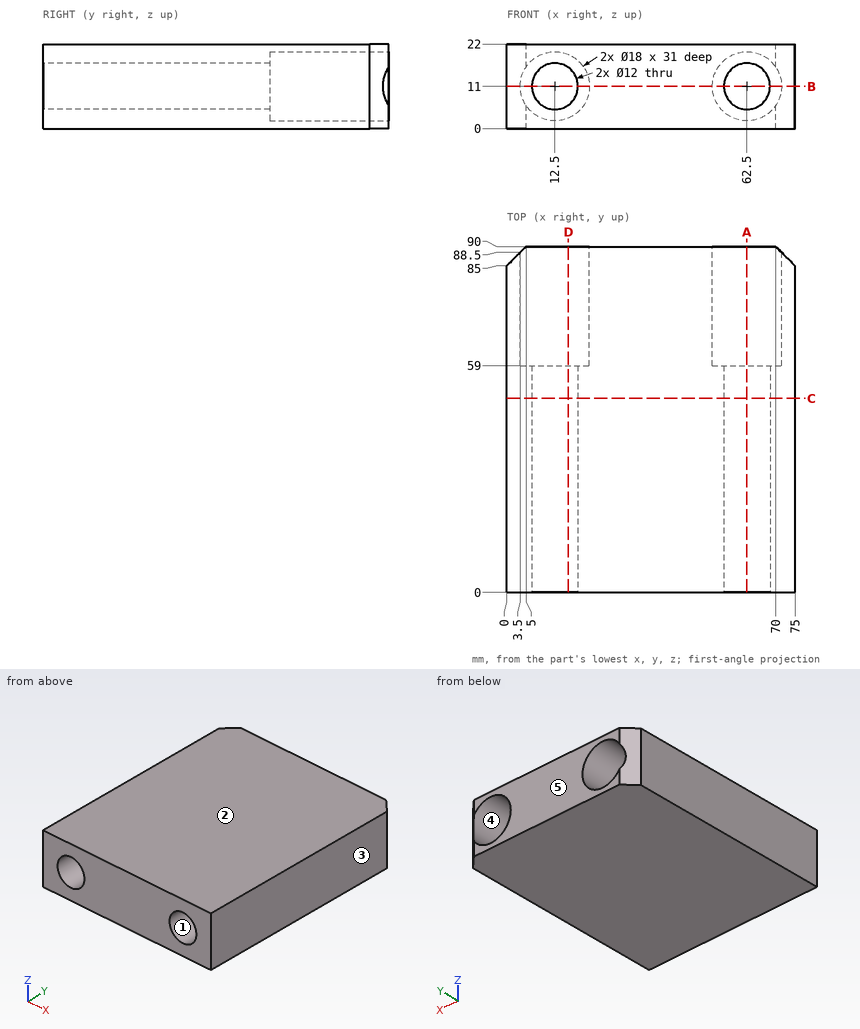
Design review of the part shown in the three views and the two pictorial views. Dimensions are in mm from the part's minimum x, y and z. A direction names the side the tool comes from. Round coordinates to 2 decimals unless told otherwise and drop trailing zeros. Write each loop counter-clockwise with the first axis right and the second up, starting at its lowest first coordinate (ties: lowest second). Pieces come first, ordered by that corner, then holes. Notation, with made-up numbers: (24, -18) - (49, -18) arc R35 cw to (49, 15) - close; hole circle Ø9 at (-17.5, 40). An arc over 180 degrees is marked (long way). Write item = value, one per line. Start each with the question number.
1. For pin 1 Ø7 at (x, z) = (62.5, 11) entering from +Y; pin 2 Ø9 at (x, z) = (11, 13.5) entering from +Y, all flat-tipped, find the tip position at first contact; note any pin that passes through.
2. Consider section A-A on x = 62.5. State the section outline as (y, z) points.
3. For the marked faces 4 and 5, list the 3-axis set-ups (+Z, -Z, +X, -X, +Y, -Y) from which the entire face can be reached by the end or side of a thin tool; tool diameter is ignored.
4. Consider section C-C on y = 50.5. State the section outline as (x, z) points, plus the area to 3 significant figures.
5. Wall thickness on L1, parallel to X at y = 25, z = 10.75; L2, parallel to X at y = 78, z = 11; L3, parallel to Z at x = 62, y = 36: over which ranges is each line inside the solid? List them lowest first.
6. Draft analysis for pull direction X (two halves, no side actions). For the marked faces 1, 2 and 3, state which applies: released by +X, released by -X, zero draft, split by the parting line, or undercut.
7. Consider section D-D on x = 16. State the section outline as (y, z) points.
8. Consider section B-B on z = 11. State the section outline as (x, y) points, plus the area to 3 significant figures.
Evaluation:
q1.pin_1 = through
q1.pin_2 = 59
q2.outline = (0, 0) - (90, 0) - (90, 2) - (59, 2) - (59, 5) - (0, 5) - close; (0, 17) - (59, 17) - (59, 20) - (90, 20) - (90, 22) - (0, 22) - close
q3.face_4 = +Y
q3.face_5 = +Z, -Z, +X, -X, +Y
q4.outline = (0, 0) - (75, 0) - (75, 22) - (0, 22) - close; hole circle Ø12 at (12.5, 11); hole circle Ø12 at (62.5, 11)
q4.area = 1,420 mm2
q5.L1 = 0 to 6.51, 18.49 to 56.51, 68.49 to 75
q5.L2 = 0 to 3.5, 21.5 to 53.5, 71.5 to 75
q5.L3 = 0 to 5.02, 16.98 to 22
q6.face_1 = undercut
q6.face_2 = zero draft
q6.face_3 = released by +X
q7.outline = (0, 0) - (90, 0) - (90, 2.71) - (59, 2.71) - (59, 6.13) - (0, 6.13) - close; (0, 15.87) - (59, 15.87) - (59, 19.29) - (90, 19.29) - (90, 22) - (0, 22) - close
q8.outline = (0, 0) - (6.5, 0) - (6.5, 59) - (3.5, 59) - (3.5, 88.5) - (0, 85) - close; (18.5, 0) - (56.5, 0) - (56.5, 59) - (53.5, 59) - (53.5, 90) - (21.5, 90) - (21.5, 59) - (18.5, 59) - close; (68.5, 0) - (75, 0) - (75, 85) - (71.5, 88.5) - (71.5, 59) - (68.5, 59) - close
q8.area = 4,200 mm2
